Source: CAD feature listing. Evaluate the final solid. Frame: model axes, mm. A direction names the side the tool comes from. Round coordinates to 2 decimals unless told otherwise and drop trailing zeros. Write each loop counter-clockwise with the first axis right and the second up, starting at its lowest first coordinate (ties: lowest second). Pieces come first, ordered by that corner, then holes. Notation, with made-up numbers: (61, 33) -> (81, 33) arc R23 ccw to (81, 42) -> close; hole circle Ø8 at (50, 73.25). An arc over 180 degrees is marked (long way). Return JSON: item names as keys, results as strings. Group by question number.
from build123d import *

# Parameters (mm, degrees)
SKETCH_2_W               = 1.6
SKETCH_2_H               = 2
CUT_EXTRUDE_1_DEPTH      = 14.5
CUT_EXTRUDE_1_DEPTH_BACK = 14.5


with BuildPart() as part:
    # Эскиз1 → Повернуть1 (revolve)
    with BuildSketch(Plane.XY):
        Polygon((-31.5, 0), (31.5, 0), (31.5, 13.5), (29.5, 13.5), (29.5, 10), (27.5, 10), (24, 13.5), (7, 13.5), (3.5, 10), (-1.5, 10), (-1.5, 7), (-13.5, 5.8), (-16, 4.5), (-17, 5.5), (-31.5, 5.5), align=None)
    revolve(axis=Axis((-261.918227013, 0, 0), (1, 0, 0)))

    # Эскиз2 → Вырез-Вытянуть1 (cut, two sides)
    with BuildSketch(Plane(origin=(0, 0, 0), x_dir=(1, 0, 0), z_dir=(0, 1, 0))) as cut_extrude_1_sk:
        with Locations((30.7, 0)):
            Rectangle(SKETCH_2_W, SKETCH_2_H)
    extrude(amount=CUT_EXTRUDE_1_DEPTH, mode=Mode.SUBTRACT)
    extrude(cut_extrude_1_sk.sketch, amount=-CUT_EXTRUDE_1_DEPTH_BACK, mode=Mode.SUBTRACT)


solid = part.part
Item 1: Cut plane B-B on z = 0. Output: boundary loops of the cut face in (x, y).
Item 2: Cut plane D-D on x = -19.5. Output: boundary loops of the cut face in (y, z).
Item 3: Set-up query: faces 1 (the cylindrical face through (15.38, -2.93, -13.18)), 2 (the flat face through (31, 0, 1)), 3 (the cylindrical face through (28.49, -2.17, -9.76)), 4 (the cylindrical face through (-24.35, -1.19, -5.37)). Return all of +Z, -Z, +X, -X, +Y, -Y with unobstructed straight access to the full face (end or side cutting, diameter ignored); none if empty.
Item 4: Cut plane C-C on x = -10.5. Output: boundary loops of the cut face in (y, z).
Item 5: Pull-direction query (X, two-part tool) for faces 5 (the flat face through (29.5, -9, -5)), 6 (the conical face through (27.28, 9.75, 3.07)), 7 (the flat face through (31.5, 0, -6)), 8 (the flat face through (31, 0, -1)); classes: +X half, -X half, draft (parallel to the pull), parting line (faces both ways), or undercut.
Item 6: Material intervals for probe 1 along Z at (x, y) = (3, 0.25); probe 2 along X at (y, z) = (-1.5, 9.5); probe 3 along X at (y, z) = (-4, -10), sorted ascending.
Item 7: First-contact query: pin 1 Ø1.3 at (x, y) = (30.5, -3) entering from +Z; pin 2 Ø10 at (x, z) = (17.5, 6.5) entering from +Y; pin 3 Ø8 at (x, z) = (-11.5, 9.5) entering from -Y. Flat tips, straight axial feed; report the tip coordinate or a pass-through.
Here are the results:
{
 "1": {"outline": "(-31.5, -5.5) -> (-17, -5.5) -> (-16, -4.5) -> (-13.5, -5.8) -> (-1.5, -7) -> (-1.5, -10) -> (3.5, -10) -> (7, -13.5) -> (24, -13.5) -> (27.5, -10) -> (29.5, -10) -> (29.5, -13.5) -> (29.9, -13.5) -> (29.9, 13.5) -> (29.5, 13.5) -> (29.5, 10) -> (27.5, 10) -> (24, 13.5) -> (7, 13.5) -> (3.5, 10) -> (-1.5, 10) -> (-1.5, 7) -> (-13.5, 5.8) -> (-16, 4.5) -> (-17, 5.5) -> (-31.5, 5.5) -> close"},
 "2": {"outline": "circle Ø11 at (0, 0)"},
 "3": {"face 1": "+X, -X", "face 2": "+X, +Y, -Y", "face 3": "none", "face 4": "-X"},
 "4": {"outline": "circle Ø12.2 at (0, 0)"},
 "5": {"face 5": "undercut", "face 6": "undercut", "face 7": "+X half", "face 8": "draft"},
 "6": {"probe 1": "z = -10 to 10", "probe 2": "x = -1.5 to 31.5", "probe 3": "x = 4.27 to 26.73, 29.5 to 31.5"},
 "7": {"pin 1": "stops at z = 13.29", "pin 2": "stops at y = 13.42", "pin 3": "stops at y = -2.45"}
}
